Geometry check sheet. Reference: the model listing, model coordinates, mm. Face numbers are marked on the shaded views. A direction names the side the tool comes from. Give positions to 0.01 mm unless a question says otherwise; leave off trailing zeros. Write each loop counter-clockwise with the first axis right and the second up, starting at its lowest first coordinate (ties: lowest second). Pieces come first, ordered by that corner, then holes.
(1) Depth check by flat-ended pin: P1, Ø2, axis at x = -25.5, y = 5.5, coming from the +Z side; P2, Ø4, axis at x = -23, y = 5.5, coming from the -Z side; P3, Ø4.5, axis at x = -0.5, z = -5, coming from the +Y side. Enter the tip coordinate at first touch or a pass-through.
(2) Cross-section at B-B (y = -13). Record the boundary of the cut face in (x, z).
(3) Cross-section at A-A (x = -41.5). Record the boundary of the cut face in (y, z), and give its area (3 significant figures).
(4) Mould release check, pull along X, two halves, no side actions. Record for the marked faces 3 and 4: +X half, -X half, draft (parallel to the pull), parting line (faces both ways), or undercut.
(5) Tool access check on the marked faces 1 and 2. Record the directions out of +Z, -Z, +X, -X, +Y, -Y that give a thin tool (end or side, any length) a straight path to the whole face; none if there is none.
(6) Cross-section at C-C (x = -21.5). Record the boundary of the cut face in (y, z), and give its area (3 significant figures).
(7) Thickness scan on line 1 along Z through (x, y) = (20, -19.5); line 2 along Z through (x, y) = (-46.5, -28.5); line 3 along Y through (x, z) = (21, 1.75). Record the ranges inside material, lowest first.
(8) Cross-section at D-D (z = -2.75). Record the boundary of the cut face in (x, y), and give its area (3 significant figures).
```python
from build123d import *

# Parameters (mm, degrees)
SKETCH_1_W          = 105.5
SKETCH_1_H          = 67.3
EXTRUDE_1_DEPTH     = 3
SKETCH_2_W          = 45.5
SKETCH_2_H          = 10.549345268
EXTRUDE_2_DEPTH     = 0.1
SKETCH_3_W          = 98.5
SKETCH_3_H          = 57.3
CUT_EXTRUDE_1_DEPTH = 0.1


with BuildPart() as part:
    # 草图1 → 凸台-拉伸1 (new body)
    with BuildSketch(Plane.XY.offset(3)):
        Rectangle(SKETCH_1_W, SKETCH_1_H)
    extrude(amount=-EXTRUDE_1_DEPTH)

    # 草图2 → 凸台-拉伸2 (add)
    with BuildSketch(Plane.XZ.offset(33.65)):
        with Locations((-10, -3.274672634)):
            Rectangle(SKETCH_2_W, SKETCH_2_H)
    extrude(amount=EXTRUDE_2_DEPTH)

    # 草图3 → 切除-拉伸1 (cut)
    with BuildSketch(Plane.XY.offset(3)):
        with Locations((0, 2.5)):
            Rectangle(SKETCH_3_W, SKETCH_3_H)
    extrude(amount=-CUT_EXTRUDE_1_DEPTH, mode=Mode.SUBTRACT)


solid = part.part
```
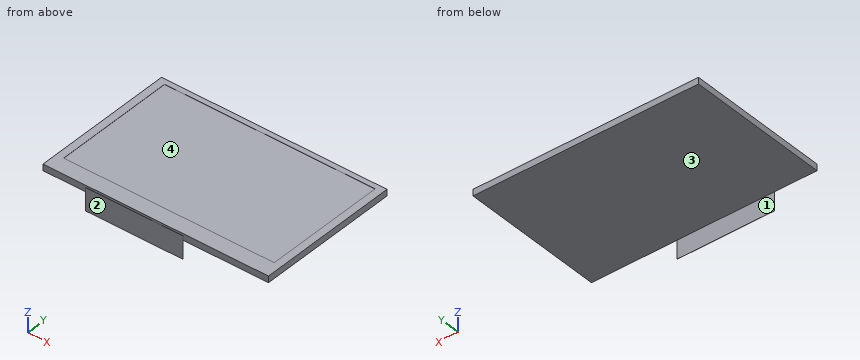
Reply:
1. P1: stops at z = 2.9
1. P2: stops at z = 0
1. P3: stops at y = -33.65
2. outline: (-52.75, 0) - (52.75, 0) - (52.75, 3) - (49.25, 3) - (49.25, 2.9) - (-49.25, 2.9) - (-49.25, 3) - (-52.75, 3) - close
3. outline: (-33.65, 0) - (33.65, 0) - (33.65, 3) - (31.15, 3) - (31.15, 2.9) - (-26.15, 2.9) - (-26.15, 3) - (-33.65, 3) - close
3. area: 196 mm2
4. face 3: draft
4. face 4: undercut
5. face 1: -Z, +X, -X, +Y
5. face 2: +Z, -Z, +X, -X, -Y
6. outline: (-33.75, -8.55) - (-33.65, -8.55) - (-33.65, 0) - (33.65, 0) - (33.65, 3) - (31.15, 3) - (31.15, 2.9) - (-26.15, 2.9) - (-26.15, 3) - (-33.65, 3) - (-33.65, 2) - (-33.75, 2) - close
6. area: 197 mm2
7. line 1: z = 0 to 2.9
7. line 2: z = 0 to 3
7. line 3: y = -33.65 to 33.65
8. outline: (-32.75, -33.75) - (12.75, -33.75) - (12.75, -33.65) - (-32.75, -33.65) - close
8. area: 4.55 mm2
